```python
from build123d import *

# Parameters (mm, degrees)
BOSS_EXTRUDE1_DEPTH = 12.7
BOSS_EXTRUDE2_DEPTH = 12.7
SKETCH18_R          = 3.175
CUT_EXTRUDE1_DEPTH  = 34.29


with BuildPart() as part:
    # Sketch1 → Boss-Extrude1 (new body)
    with BuildSketch(Plane.XY):
        with BuildLine():
            Line((36.21435187, 2.127742376), (36.21435187, -23.272257624))
            Line((36.21435187, -23.272257624), (-36.21435187, -23.272257624))
            Line((-36.21435187, -23.272257624), (-36.21435187, 2.127742376))
            Line((-36.21435187, 2.127742376), (-20.97435187, 2.127742376))
            ThreePointArc((-20.97435187, 2.127742376), (0, -21.082), (20.97435187, 2.127742376))
            Line((20.97435187, 2.127742376), (36.21435187, 2.127742376))
        make_face()
    extrude(amount=BOSS_EXTRUDE1_DEPTH)

    # Sketch3 → Boss-Extrude2 (add)
    with BuildSketch(Plane.XY):
        with BuildLine():
            Line((-20.97435187, 2.127742376), (-36.21435187, 2.127742376))
            Line((-36.21435187, 2.127742376), (-36.21435187, 11.017742376))
            Line((-36.21435187, 11.017742376), (-23.036618604, 11.017742376))
            ThreePointArc((-23.036618604, 11.017742376), (0, 25.535787511), (23.036618604, 11.017742376))
            Line((23.036618604, 11.017742376), (36.279630177, 11.017742376))
            Line((36.279630177, 11.017742376), (36.279630177, 2.127742376))
            Line((36.279630177, 2.127742376), (20.97435187, 2.127742376))
            ThreePointArc((20.97435187, 2.127742376), (0, 21.082), (-20.97435187, 2.127742376))
        make_face()
    extrude(amount=BOSS_EXTRUDE2_DEPTH)

    # Sketch18 → Cut-Extrude1 (cut)
    with BuildSketch(Plane(origin=(0, 11.017742376, 0), x_dir=(1, 0, 0), z_dir=(0, 1, 0))):
        with Locations(Location((-29.658124391, -6.35, 0), (0, 0, 180))):
            Circle(SKETCH18_R)
        with Locations(Location((29.658124391, -6.35, 0), (0, 0, 180))):
            Circle(SKETCH18_R)
    extrude(amount=-CUT_EXTRUDE1_DEPTH, mode=Mode.SUBTRACT)


solid = part.part
```
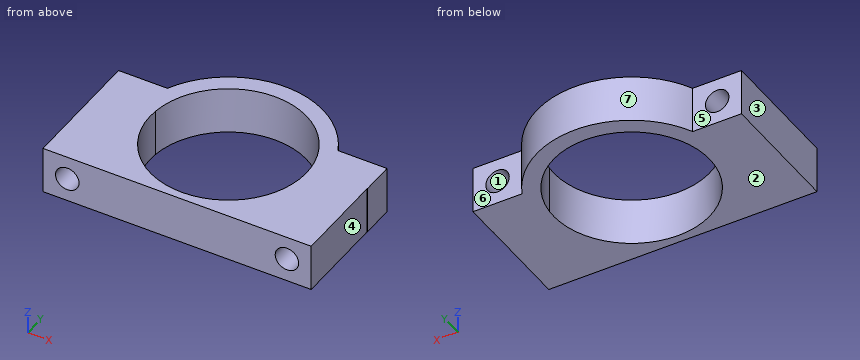
The model under review builds one solid part; all positions refer to its coordinate system, in mm. Face numbers are marked on the shaded views. A direction names the side the tool comes from. Coordinates: 2 decimals unless noted, no trailing zeros. Write each loop counter-clockwise with the first axis right and the second up, starting at its lowest first coordinate (ties: lowest second). Pieces come first, ordered by that corner, then holes. Notation, with made-up numbers: (-26.5, 8.25) - (32.5, 8.25) arc R33 cw to (32.5, 41.25) - close; hole circle Ø6 at (-13, 54.5). An arc over 180 degrees is marked (long way). Write item = value, one per line.
(1) Consider section D-D, the plane z = 11. Give the boundary of the cut face in (x, y), then the cut area to 3 significant figures.
Result sheet:
outline = (-36.21, -23.27) - (36.21, -23.27) - (36.21, 2.13) - (36.28, 2.13) - (36.28, 11.02) - (23.04, 11.02) arc R25.54 ccw to (-23.04, 11.02) - (-36.21, 11.02) - close; hole circle Ø42.16 at (0, 0)
area = 1,570 mm^2
(2) For line 1 (Y direction, x = 0.5, z = 11.25); line 2 (X direction, y = -5, z = 4); line 3 (X direction, y = 4.5, z = 7), list the stretches that pass through material, from the lowest coordinate up. Write a range as [from, to].
Result sheet:
line_1 = [-23.27, -21.08], [21.08, 25.53]
line_2 = [-36.21, -31.79], [-27.52, -20.48], [20.48, 27.52], [31.79, 36.21]
line_3 = [-36.21, -32.77], [-26.55, -20.6], [20.6, 26.55], [32.77, 36.28]
(3) Consider section A-A, the plane y = 0. Give the boundary of the cut face in (x, z) (3 decimals).
Result sheet:
outline = (-36.214, 0) - (-21.082, 0) - (-21.082, 12.7) - (-36.214, 12.7) - close; (21.082, 0) - (36.214, 0) - (36.214, 12.7) - (21.082, 12.7) - close; hole circle Ø6.35 at (-29.658, 6.35); hole circle Ø6.35 at (29.658, 6.35)
(4) For P1, Ø2, axis at x = 24, y = 3, coming from the -Z side; P2, Ø1, axis at y = -10, z = 5.5, coming from the +X side; P3, Ø5, axis at x = -15.5, z = 9, coming from the +Y side; P4, Ø2, axis at y = 19, z = 11, coming from the -X side, all flat-tipped, find the tip position at first contact; note any pin that passes through.
Result sheet:
P1 = 0
P2 = 36.21
P3 = 21.98
P4 = -18.11
(5) Machinability: for the marked faces 4, 5, 6 and 7, which of the approach directions +Z, -Z, +X, -X, +Y, -Y give a long, thin tool a straight path to every point of the face, cutting with its end or side? Answer none if there is none.
Result sheet:
face_4 = +Z, -Z, +X, -Y
face_5 = +Z, -Z, -X, +Y
face_6 = +Z, -Z, +X, +Y
face_7 = +Z, -Z, +Y
(6) Consider section C-C, the plane x = 0. Give the boundary of the cut face in (y, z), then the cut area to 3 significant figures.
Result sheet:
outline = (-23.27, 0) - (-21.08, 0) - (-21.08, 12.7) - (-23.27, 12.7) - close; (21.08, 0) - (25.54, 0) - (25.54, 12.7) - (21.08, 12.7) - close
area = 84.4 mm^2
(7) Mouldability with a two-part tool opening along Z and no side actions: class the marked faces 1, 2 and 3 as pulls with the +Z half, pulls with the -Z half, needs draft (parallel to the pull), parting line crosses it, or undercut.
Result sheet:
face_1 = undercut
face_2 = pulls with the -Z half
face_3 = needs draft
(8) Consider section B-B, the plane z = 6.35. Give the boundary of the cut face in (x, y).
Result sheet:
outline = (-36.21, -23.27) - (-32.83, -23.27) - (-32.83, 11.02) - (-36.21, 11.02) - close; (-26.48, -23.27) - (26.48, -23.27) - (26.48, 11.02) - (23.04, 11.02) arc R25.54 ccw to (-23.04, 11.02) - (-26.48, 11.02) - close; (32.83, -23.27) - (36.21, -23.27) - (36.21, 2.13) - (36.28, 2.13) - (36.28, 11.02) - (32.83, 11.02) - close; hole circle Ø42.16 at (0, 0)
